```python
from build123d import *

# Parameters (mm, degrees)
HOLE1_D                           = 30
M10X1_25_TAPPED_HOLE1_D           = 8.8
M10X1_25_TAPPED_HOLE1_CSINK_D     = 10.05
M10X1_25_TAPPED_HOLE1_CSINK_ANGLE = 90
CIRPATTERN1_COUNT                 = 3


with BuildPart() as part:
    # Sketch1 → Revolve1 (revolve)
    with BuildSketch(Plane(origin=(0, 0, 0), x_dir=(0, 0, -1), z_dir=(1, 0, 0))):
        Polygon((0, 0), (0, 24), (25, 24), (25, 12), (53, 12), (53, 0), align=None)
    revolve(axis=Axis((0, 0, 0), (0, 1, 0)))

    # Hole1 (through all)
    with Locations(Plane(origin=(0, 24, 0), x_dir=(1, 0, 0), z_dir=(0, 1, 0))):
        with Locations((0, 0)):
            Hole(HOLE1_D / 2)

    # M10x1.25 Tapped Hole1 (through all)
    with Locations(Plane(origin=(0, 12, 0), x_dir=(1, 0, 0), z_dir=(0, 1, 0))):
        with Locations((0, 37.5)):
            m10x1_25_tapped_hole1 = CounterSinkHole(M10X1_25_TAPPED_HOLE1_D / 2, M10X1_25_TAPPED_HOLE1_CSINK_D / 2, counter_sink_angle=M10X1_25_TAPPED_HOLE1_CSINK_ANGLE)

    # CirPattern1: M10x1.25 Tapped Hole1 ×3 about axis
    cirpattern1_axis = Axis((0, 0, 0), (0, 1, 0))
    for i in range(1, CIRPATTERN1_COUNT):
        add(m10x1_25_tapped_hole1.rotate(cirpattern1_axis, i * 360 / CIRPATTERN1_COUNT), mode=Mode.SUBTRACT)


solid = part.part
```
Input: part model. Units: mm. Frame: model coordinates. A direction names the side the tool comes from. Coordinates: 2 decimals unless noted, no trailing zeros. Loops run counter-clockwise (first coordinate to the right, second up) from the corner with the lowest first, then second, coordinate; pieces in that order, holes last. Notation, with made-up numbers: M 29,83.25 L 85,83.25 A30 ccw 85,113.25 Z; hole C 27,-27.5 d6. An arc over 180 degrees is marked long. Answer in a Markdown table with one row per item.
1. Section C-C, the plane x = -11. Output: boundary loops of the cut face in (y, z), then the cut area to 3 significant figures.
Response:
| item | result |
|---|---|
| outline | M 0,-51.85 L 12,-51.85 L 12,-22.45 L 24,-22.45 L 24,-10.2 L 0,-10.2 Z; M 0,10.2 L 24,10.2 L 24,22.45 L 12,22.45 L 12,51.85 L 0,51.85 Z |
| area | 1,290 mm2 |
2. Section A-A, the plane x = 0. Output: boundary loops of the cut face in (y, z) (3 decimals), then the cut area to 3 significant figures.
Response:
| item | result |
|---|---|
| outline | M 0,-53 L 12,-53 L 12,-42.525 L 11.375,-41.9 L 0,-41.9 Z; M 0,-33.1 L 11.375,-33.1 L 12,-32.475 L 12,-25 L 24,-25 L 24,-15 L 0,-15 Z; M 0,15 L 24,15 L 24,25 L 12,25 L 12,53 L 0,53 Z |
| area | 1,050 mm2 |
3. First-contact query: pin 1 (6 mm diameter, centred on y = 5, z = -12.5, fed in from +X); pin 2 (8 mm diameter, centred on x = -29.5, y = 19.5, fed in from +Z); pin 3 (8 mm diameter, centred on x = -23.5, y = 19.5, fed in from +Z); pin 4 (1 mm diameter, centred on y = 5.5, z = -0.5, fed in from +X). Flat tips, straight axial feed; report the tip coordinate or a pass-through.
Response:
| item | result |
|---|---|
| pin 1 | stops at x = 52.14 |
| pin 2 | passes through |
| pin 3 | stops at z = 15.64 |
| pin 4 | stops at x = 53 |
4. Material intervals for line 1 (Z direction, x = 0, y = 7.25); line 2 (Z direction, x = 0, y = 15.75); line 3 (Y direction, x = -17, z = 19.5), sorted ascending.
Response:
| item | result |
|---|---|
| line 1 | z = -53 to -41.9, -33.1 to -15, 15 to 53 |
| line 2 | z = -25 to -15, 15 to 25 |
| line 3 | y = 0 to 12 |
5. Draft query along Z for faces 1 (the flat face through (11, 0, -11)), 2 (the cylindrical face through (-34.84, 5.61, 15.04)), 3 (the cylindrical face through (-7.509, 17.916, -23.846)). Return one class per face: pulls with the +Z half, pulls with the -Z half, needs draft (parallel to the pull), parting line crosses it, or undercut.
Response:
| item | result |
|---|---|
| face 1 | needs draft |
| face 2 | undercut |
| face 3 | parting line crosses it |
6. Reachability of faces 4 (the flat face through (11, 12, 23)), 5 (the cylindrical face through (14.985, 11.832, -0.66)) from +Z, -Z, +X, -X, +Y, -Y: full face, straight path, thin tool, end or side. Return the list, or none.
Response:
| item | result |
|---|---|
| face 4 | +Y |
| face 5 | +Y, -Y |
7. Section D-D, the plane z = -23. Output: boundary loops of the cut face in (x, y).
Response:
| item | result |
|---|---|
| outline | M -47.75,0 L 47.75,0 L 47.75,12 L 9.8,12 L 9.8,24 L -9.8,24 L -9.8,12 L -47.75,12 Z |
8. Section B-B, the plane z = 0. Output: boundary loops of the cut face in (x, y).
Response:
| item | result |
|---|---|
| outline | M -53,0 L -15,0 L -15,24 L -25,24 L -25,12 L -53,12 Z; M 15,0 L 53,0 L 53,12 L 25,12 L 25,24 L 15,24 Z |
